Design review of the part built by this model. Coordinates are the model's own, in mm. A direction names the side the tool comes from. Coordinates: 2 decimals unless noted, no trailing zeros. Write each loop counter-clockwise with the first axis right and the second up, starting at its lowest first coordinate (ties: lowest second). Pieces come first, ordered by that corner, then holes. Notation, with made-up numbers: (-16, 62.25) - (35, 62.25) arc R13 ccw to (35, 81.25) - close; hole circle Ø1 at (37, 15). An arc over 180 degrees is marked (long way). Answer as CSV lines item,"result". Start each with the question number.
Q1. Machinability: for faces 1 (the face through (32.538, 20, 2)), 2 (the face through (54, -17.5, 2)), 3 (the face through (42.387, 20, 2)), 4 (the face through (-19, -17.5, 2)), which of the approach directions +Z, -Z, +X, -X, +Y, -Y give a long, thin tool a straight path to every point of the face, cutting with its end or side? Answer none if there is none.
Q2. We need section A-A (y = -19). Write out the cut boundary in (x, z) (1 decimal), plus the area to 3 significant figures.
Q3. We need section C-C (x = -28). Write out the cut boundary in (y, z).
Q4. Clearance check with flat-ended pins moving along their axes: pin 1 (1.5 mm diameter, centred on y = 18.5, z = 2.5, fed in from +X); pin 2 (1.5 mm diameter, centred on x = 53.5, z = 2, fed in from -Y); pin 3 (4 mm diameter, centred on x = 48.5, y = -5.5, fed in from -Z); pin 4 (1.5 mm diameter, centred on y = 6, z = 2, fed in from -X). State where each tip first meets the part, or that it passes through.
Q5. For line 1 along X through (y, z) = (-20, 3.6) (1 decimal); line 2 along X through (y, z) = (16, 2.3) (1 decimal); line 3 along X through (y, z) = (5.5, 0.4), list the stretches that pass through material, from the lowest coordinate up. Write a range as [from, to].
Q6. We need section D-D (y = -10). Write out the cut boundary in (x, z), plus the area to 3 significant figures.
from build123d import *

# Parameters (mm, degrees)
SKETCH2_W           = 130
SKETCH2_H           = 35
SKETCH2_W_2         = 5
SKETCH2_H_2         = 17.475
SKETCH2_W_3         = 9.85
SKETCH2_H_3         = 5
BOSS_EXTRUDE1_DEPTH = 5
SKETCH3_W           = 27.6125
SKETCH3_H           = 10
CUT_EXTRUDE1_DEPTH  = 74.697014865


with BuildPart() as part:
    # Sketch2 → Boss-Extrude1 (new body)
    with BuildSketch(Plane.XY):
        Rectangle(SKETCH2_W, SKETCH2_H)
        with Locations((-67.5, -8.7625)):
            Rectangle(SKETCH2_W_2, SKETCH2_H_2)
        with Locations((-37.4625, 20)):
            Rectangle(SKETCH2_W_3, SKETCH2_H_3)
        with Locations((0, 20)):
            Rectangle(SKETCH2_W_3, SKETCH2_H_3)
        with Locations((37.4625, 20)):
            Rectangle(SKETCH2_W_3, SKETCH2_H_3)
        with Locations((67.5, 8.7625)):
            Rectangle(SKETCH2_W_2, SKETCH2_H_2)
        with Locations((37.4625, -20)):
            Rectangle(SKETCH2_W_3, SKETCH2_H_3)
        with Locations((0, -20)):
            Rectangle(SKETCH2_W_3, SKETCH2_H_3)
        with Locations((-37.4625, -20)):
            Rectangle(SKETCH2_W_3, SKETCH2_H_3)
    extrude(amount=BOSS_EXTRUDE1_DEPTH)

    # Sketch3 → Cut-Extrude1 (cut, through all)
    with BuildSketch(Plane(origin=(0, 0, 0), x_dir=(-1, 0, 0), z_dir=(0, 0, -1))):
        with Locations((18.73125, 12.5)):
            Rectangle(SKETCH3_W, SKETCH3_H)
    extrude(amount=-CUT_EXTRUDE1_DEPTH, mode=Mode.SUBTRACT)


solid = part.part
Results list:
1,face 1,"+Z, -Z, +Y"
1,face 2,"+Z, -Z, +X, -Y"
1,face 3,"+Z, -Z, +X, +Y"
1,face 4,"+Z, -Z, -Y"
2,outline,"(-42.4, 0) - (-32.5, 0) - (-32.5, 5) - (-42.4, 5) - close; (-4.9, 0) - (4.9, 0) - (4.9, 5) - (-4.9, 5) - close; (32.5, 0) - (42.4, 0) - (42.4, 5) - (32.5, 5) - close"
2,area,"148 mm2"
3,outline,"(-17.5, 0) - (7.5, 0) - (7.5, 5) - (-17.5, 5) - close"
4,pin 1,"stops at x = 42.39"
4,pin 2,"stops at y = -17.5"
4,pin 3,"stops at z = 0"
4,pin 4,"stops at x = -65"
5,line 1,"x = [-42.4, -32.5], [-4.9, 4.9], [32.5, 42.4]"
5,line 2,"x = [-65, -32.5], [-4.9, 70]"
5,line 3,"x = [-65, 70]"
6,outline,"(-70, 0) - (65, 0) - (65, 5) - (-70, 5) - close"
6,area,"675 mm2"
